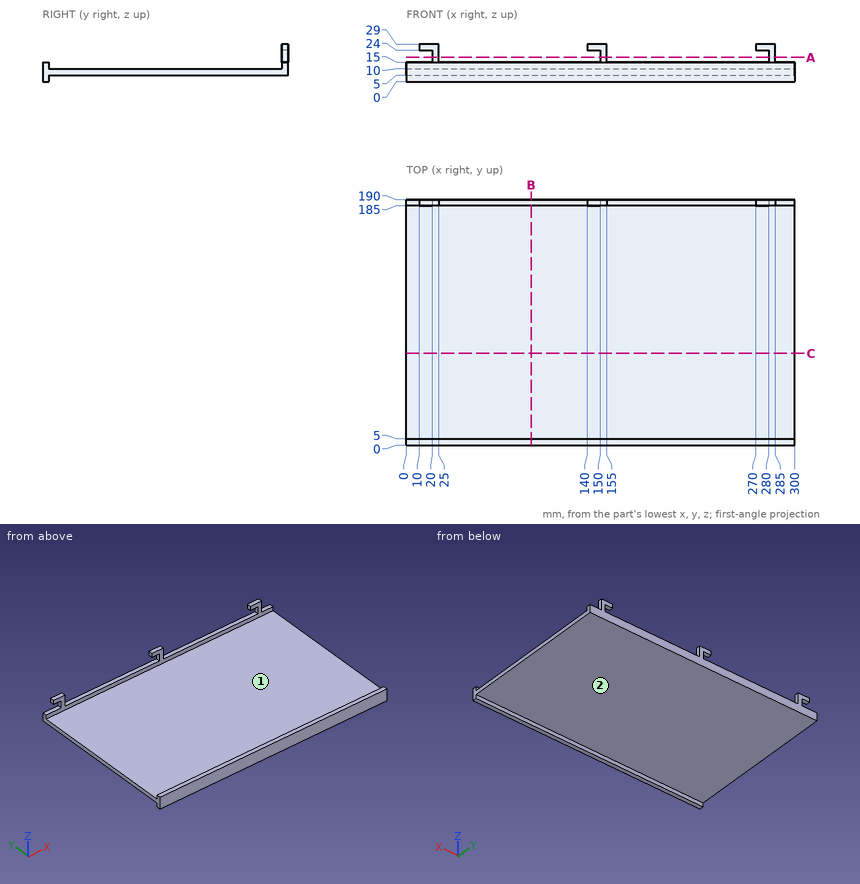
Input: dimensioned drawing with shaded views. Units: mm. Origin: part minimum x, y, z. A direction names the side the tool comes from. Coordinates: 2 decimals unless noted, no trailing zeros. Write each loop counter-clockwise with the first axis right and the second up, starting at its lowest first coordinate (ties: lowest second). Pieces come first, ordered by that corner, then holes. Notation, with made-up numbers: M 2.25,-7.5 L 19.25,-7.5 A27 cw 19.25,17.5 Z; hole C 56.5,6 d4. An arc over 180 degrees is marked long. Answer as a JSON object with one key per item and string values. Group by question number.
(1) Section C-C on y = 71. Output: boundary loops of the cut face in (x, z), plus the area to 3 significant figures.
(2) Section B-B on x = 96.5. Output: boundary loops of the cut face in (y, z).
(3) Ray query, line 1 along Y through (x, z) = (134, 13); line 2 along Z through (x, y) = (108.5, 127); line 3 along Y through (x, z) = (284.5, 21.5). Return the intervals inside material, ascending. Write a range as [from, to].
(4) Set-up query: the marked faces 1 and 2. Return all of +Z, -Z, +X, -X, +Y, -Y with unobstructed straight access to the full face (end or side cutting, diameter ignored); none if empty.
(5) Contact query for flat-ended pins moving along their axis: P1, Ø4, axis at y = 120.5, z = 8, coming from the -X side; P2, Ø5.5, axis at y = 186.5, z = 23.5, coming from the +X side; P3, Ø1.5, axis at x = 119.5, z = 3, coming from the +Y side; P4, Ø1.5, axis at x = 225, y = 186.5, coming from the +Z side. Output: stop coordinate, or through.
(6) Section A-A on z = 18.75. Output: boundary loops of the cut face in (x, y), plus the area to 3 significant figures.
Result set:
{
 "1": {"outline": "M 0,5 L 300,5 L 300,10 L 0,10 Z", "area": "1,500 mm2"},
 "2": {"outline": "M 0,0 L 5,0 L 5,5 L 190,5 L 190,15 L 185,15 L 185,10 L 5,10 L 5,15 L 0,15 Z"},
 "3": {"line 1": "y = [0, 5], [185, 190]", "line 2": "z = [5, 10]", "line 3": "y = [185, 190]"},
 "4": {"face 1": "+Z, +X, -X", "face 2": "-Z, +X, -X, +Y"},
 "5": {"P1": "stops at x = 0", "P2": "stops at x = 285", "P3": "stops at y = 5", "P4": "stops at z = 15"},
 "6": {"outline": "M 20,185 L 25,185 L 25,190 L 20,190 Z; M 150,185 L 155,185 L 155,190 L 150,190 Z; M 280,185 L 285,185 L 285,190 L 280,190 Z", "area": "75.0 mm2"}
}
